```python
from build123d import *

# Parameters (mm, degrees)
CROQUIS1_R              = 10
CROQUIS1_R_2            = 3.5
EXTRUIR1_DEPTH          = 12
CROQUIS2_W              = 45
CROQUIS2_H              = 22
SALIENTE_EXTRUIR1_DEPTH = 5
REDONDEO1_R             = 5
REDONDEO2_R             = 5
REDONDEO3_R             = 5
REDONDEO4_R             = 5
CROQUIS3_R              = 4.1
CORTAR_EXTRUIR1_DEPTH   = 45
CROQUIS4_R              = 1.55
CORTAR_EXTRUIR2_DEPTH   = 45


with BuildPart() as part:
    # Croquis1 → Extruir1 (new body)
    with BuildSketch(Plane(origin=(0, 0, 0), x_dir=(1, 0, 0), z_dir=(0, 1, 0))):
        Circle(CROQUIS1_R)
        Circle(CROQUIS1_R_2, mode=Mode.SUBTRACT)
    extrude(amount=EXTRUIR1_DEPTH)

    # Croquis2 → Saliente-Extruir1 (add)
    with BuildSketch(Plane(origin=(0, 12, 0), x_dir=(1, 0, 0), z_dir=(0, 1, 0))):
        Rectangle(CROQUIS2_W, CROQUIS2_H)
    extrude(amount=SALIENTE_EXTRUIR1_DEPTH)

    # Redondeo1
    redondeo1_edges = [part.edges().sort_by_distance(p)[0] for p in [
        (22.5, 14.5, -11),
    ]]
    fillet(redondeo1_edges, radius=REDONDEO1_R)

    # Redondeo2
    redondeo2_edges = [part.edges().sort_by_distance(p)[0] for p in [
        (22.5, 14.5, 11),
    ]]
    fillet(redondeo2_edges, radius=REDONDEO2_R)

    # Redondeo3
    redondeo3_edges = [part.edges().sort_by_distance(p)[0] for p in [
        (-22.5, 14.5, 11),
    ]]
    fillet(redondeo3_edges, radius=REDONDEO3_R)

    # Redondeo4
    redondeo4_edges = [part.edges().sort_by_distance(p)[0] for p in [
        (-22.5, 14.5, -11),
    ]]
    fillet(redondeo4_edges, radius=REDONDEO4_R)

    # Croquis3 → Cortar-Extruir1 (cut)
    with BuildSketch(Plane.XZ):
        Circle(CROQUIS3_R)
    extrude(amount=-CORTAR_EXTRUIR1_DEPTH, mode=Mode.SUBTRACT)

    # Croquis4 → Cortar-Extruir2 (cut)
    with BuildSketch(Plane.XZ.offset(-12)):
        with Locations((-16.5, 5)):
            Circle(CROQUIS4_R)
        with Locations((-16.5, -5)):
            Circle(CROQUIS4_R)
        with Locations((16.5, 5)):
            Circle(CROQUIS4_R)
        with Locations((16.5, -5)):
            Circle(CROQUIS4_R)
    extrude(amount=-CORTAR_EXTRUIR2_DEPTH, mode=Mode.SUBTRACT)


solid = part.part
```
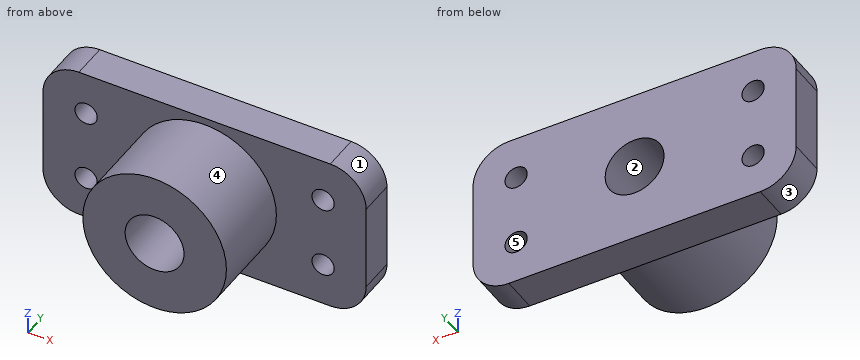
For this review, take the finished solid that the model builds, in its own axes (mm). Face numbers are marked on the shaded views. A direction names the side the tool comes from. Round coordinates to 2 decimals unless told otherwise and drop trailing zeros. Order: outer loops, then holes, each group sorted by start corner. A loop starts at its lowest first (then second) coordinate and runs counter-clockwise, first axis right, second up.
Q1. We need section C-C, the plane x = 16.5. Give the boundary of the cut face in (y, z), plus the area to 3 significant figures.
Findings below:
outline: (12, -11) - (17, -11) - (17, -6.55) - (12, -6.55) - close; (12, -3.45) - (17, -3.45) - (17, 3.45) - (12, 3.45) - close; (12, 6.55) - (17, 6.55) - (17, 11) - (12, 11) - close
area: 79.0 mm2
Q2. We need section D-D, the plane y = 8.75. Give the boundary of the cut face in (x, z), plus the area to 3 significant figures.
Findings below:
outline: circle Ø20 at (0, 0); hole circle Ø8.2 at (0, 0)
area: 261 mm2
Q3. Wall thickness on line 1 (Z direction, x = -16.5, y = 14.5); line 2 (Y direction, x = -11.5, z = 3.5); line 3 (X direction, y = 2.5, z = 1.75): over which ranges is each line inside the solid? List them lowest first.
Findings below:
line 1: z = -11 to -6.55, -3.45 to 3.45, 6.55 to 11
line 2: y = 12 to 17
line 3: x = -9.85 to -3.71, 3.71 to 9.85
Q4. We need section B-B, the plane z = 0. Give the boundary of the cut face in (x, y).
Findings below:
outline: (-22.5, 12) - (-10, 12) - (-10, 0) - (-4.1, 0) - (-4.1, 17) - (-22.5, 17) - close; (4.1, 0) - (10, 0) - (10, 12) - (22.5, 12) - (22.5, 17) - (4.1, 17) - close
Q5. We need section A-A, the plane x = 0. Give the boundary of the cut face in (y, z), plus the area to 3 significant figures.
Findings below:
outline: (0, -10) - (12, -10) - (12, -11) - (17, -11) - (17, -4.1) - (0, -4.1) - close; (0, 4.1) - (17, 4.1) - (17, 11) - (12, 11) - (12, 10) - (0, 10) - close
area: 211 mm2
Q6. Insertion check: P1, Ø3.5, axis at x = -16.5, z = 5, coming from the -Y side; P2, Ø6, axis at x = 8.5, y = 5.5, coming from the -Z side; P3, Ø5, axis at y = 8.5, z = -5.5, coming from the -X side. Each pin has a flat end and moves straight along its axis. Give the tip position at first contact, or say it passes through.
Findings below:
P1: stops at y = 12
P2: stops at z = -8.35
P3: stops at x = -9.54
Q7. Mouldability with a two-part tool opening along X and no side actions: class the marked faces 1, 2 and 3 as pulls with the +X half, pulls with the -X half, needs draft (parallel to the pull), parting line crosses it, or undercut.
Findings below:
face 1: pulls with the +X half
face 2: undercut
face 3: pulls with the -X half
Q8. Machinability: for the marked faces 4 and 5, which of the approach directions +Z, -Z, +X, -X, +Y, -Y give a long, thin tool a straight path to every point of the face, cutting with its end or side? Answer none if there is none.
Findings below:
face 4: -Y
face 5: +Y, -Y
